Geometry check sheet. Reference: the model listing, model coordinates, mm. Face numbers are marked on the shaded views. A direction names the side the tool comes from. Coordinates: 2 decimals unless noted, no trailing zeros. Loops run counter-clockwise (first coordinate to the right, second up) from the corner with the lowest first, then second, coordinate; pieces in that order, holes last.
from build123d import *

# Parameters (mm, degrees)
SKETCH1_W           = 10
SKETCH1_H           = 3.18
BOSS_EXTRUDE1_DEPTH = 1.5875


with BuildPart() as part:
    # Sketch1 → Boss-Extrude1 (new, symmetric)
    with BuildSketch(Plane.XY):
        Polygon((0, 0), (0, -3.18), (-10, -3.18), (-10, 0), (-17.765, 0), (-17.765, 42.35), (-10, 42.35), (-10, 45.53), (0, 45.53), (0, 42.35), (7.765, 42.35), (7.765, 0), align=None)
        with Locations((-5, 13.586666667)):
            Rectangle(SKETCH1_W, SKETCH1_H, mode=Mode.SUBTRACT)
        with Locations((-5, 28.763333333)):
            Rectangle(SKETCH1_W, SKETCH1_H, mode=Mode.SUBTRACT)
    extrude(amount=BOSS_EXTRUDE1_DEPTH, both=True)


solid = part.part
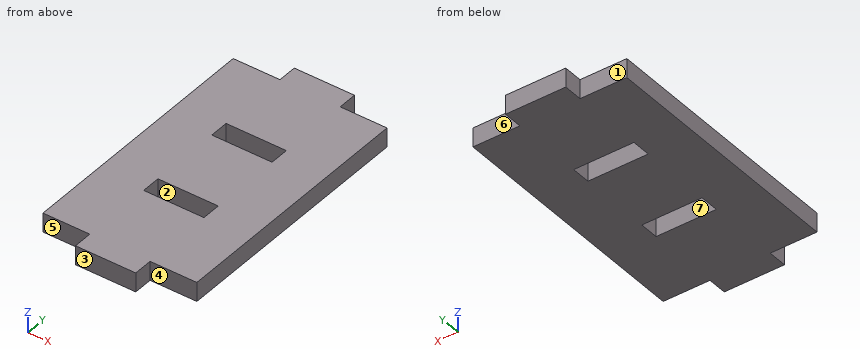
(1) Sectioned sample at D-D on x = -13.75. Record the cut outline in (y, z), and give its area (3 significant figures).
Findings:
outline: (0, -1.59) - (42.35, -1.59) - (42.35, 1.59) - (0, 1.59) - close
area: 134 mm2
(2) Draft check along X on the marked faces 1 and 2. Enter one of: +X half, -X half, draft (parallel to the pull), parting line (faces both ways), or undercut.
Findings:
face 1: draft
face 2: undercut
(3) Sectioned sample at C-C on z = -0.1. Record the cut outline in (x, y) (3 decimals).
Findings:
outline: (-17.765, 0) - (-10, 0) - (-10, -3.18) - (0, -3.18) - (0, 0) - (7.765, 0) - (7.765, 42.35) - (0, 42.35) - (0, 45.53) - (-10, 45.53) - (-10, 42.35) - (-17.765, 42.35) - close; hole (-10, 11.997) - (0, 11.997) - (0, 15.177) - (-10, 15.177) - close; hole (-10, 27.173) - (0, 27.173) - (0, 30.353) - (-10, 30.353) - close
(4) Gauge pin test, flat ends, axial feed: pin 1 Ø1.6 at (y, z) = (43.5, 0) entering from +X; pin 2 Ø1 at (y, z) = (44.5, 0) entering from -X; pin 3 Ø1 at (x, z) = (5, 0) entering from +Y. Record the tip position at first contact, or that the pin passes through.
Findings:
pin 1: stops at x = 0
pin 2: stops at x = -10
pin 3: stops at y = 42.35
(5) Access from +Z, -Z, +X, -X, +Y, -Y to the whole of each face (thin tool, end or side, straight path). Record for the marked faces 3, 4, 5, 6 and 7.
Findings:
face 3: +Z, -Z, +X, -X, -Y
face 4: +Z, -Z, +X, -Y
face 5: +Z, -Z, -X, -Y
face 6: +Z, -Z, +X, +Y
face 7: +Z, -Z
(6) Sectioned sample at B-B on x = -2.75. Record the cut outline in (y, z), and give its area (3 significant figures).
Findings:
outline: (-3.18, -1.59) - (12, -1.59) - (12, 1.59) - (-3.18, 1.59) - close; (15.18, -1.59) - (27.17, -1.59) - (27.17, 1.59) - (15.18, 1.59) - close; (30.35, -1.59) - (45.53, -1.59) - (45.53, 1.59) - (30.35, 1.59) - close
area: 134 mm2
(7) Sectioned sample at A-A on y = 13.5. Record the cut outline in (x, z) (1 decimal), and give its area (3 significant figures).
Findings:
outline: (-17.8, -1.6) - (-10, -1.6) - (-10, 1.6) - (-17.8, 1.6) - close; (0, -1.6) - (7.8, -1.6) - (7.8, 1.6) - (0, 1.6) - close
area: 49.3 mm2
(8) Scan lines: L1, parallel to Y at x = -3.5, z = 0.25; L2, parallel to X at y = 15, z = -0.5 (3 decimals); L3, parallel to Y at x = -10.25, z = 1.2. Record each from-to range of solid material in increasing order.
Findings:
L1: y = -3.18 to 12, 15.18 to 27.17, 30.35 to 45.53
L2: x = -17.765 to -10, 0 to 7.765
L3: y = 0 to 42.35
